```python
from build123d import *

# Parameters (mm, degrees)
SKETCH1_W           = 60
SKETCH1_H           = 27
BOSS_EXTRUDE1_DEPTH = 10
SKETCH2_R           = 2.6
CUT_EXTRUDE1_DEPTH  = 42.581245773
SKETCH3_R           = 4.75
CUT_EXTRUDE2_DEPTH  = 22
SKETCH4_W           = 60
SKETCH4_H           = 7
SKETCH4_W_2         = 40
SKETCH4_H_2         = 5
BOSS_EXTRUDE3_DEPTH = 28
SKETCH5_R           = 2.6
CUT_EXTRUDE3_DEPTH  = 50.122296363
SKETCH6_R           = 1.6
CUT_EXTRUDE4_DEPTH  = 51.261814532


with BuildPart() as part:
    # Sketch1 → Boss-Extrude1 (new body)
    with BuildSketch(Plane(origin=(0, 0, 0), x_dir=(1, 0, 0), z_dir=(0, 1, 0))):
        Rectangle(SKETCH1_W, SKETCH1_H)
    extrude(amount=BOSS_EXTRUDE1_DEPTH)

    # Sketch2 → Cut-Extrude1 (cut, through all)
    with BuildSketch(Plane.XY.offset(13.5)):
        with Locations((0, 5)):
            Circle(SKETCH2_R)
    extrude(amount=-CUT_EXTRUDE1_DEPTH, mode=Mode.SUBTRACT)

    # Sketch3 → Cut-Extrude2 (cut)
    with BuildSketch(Plane.XY.offset(13.5)):
        with Locations((0, 5)):
            Circle(SKETCH3_R)
    extrude(amount=-CUT_EXTRUDE2_DEPTH, mode=Mode.SUBTRACT)

    # Sketch4 → Boss-Extrude3 (add)
    with BuildSketch(Plane.XZ):
        with Locations((0, 10)):
            Rectangle(SKETCH4_W, SKETCH4_H)
        with Locations((0, 10)):
            Rectangle(SKETCH4_W_2, SKETCH4_H_2, mode=Mode.SUBTRACT)
    extrude(amount=BOSS_EXTRUDE3_DEPTH)

    # Sketch5 → Cut-Extrude3 (cut, through all)
    with BuildSketch(Plane.XY.offset(13.5)):
        with Locations((0, -22.5)):
            Circle(SKETCH5_R)
    extrude(amount=-CUT_EXTRUDE3_DEPTH, mode=Mode.SUBTRACT)

    # Sketch6 → Cut-Extrude4 (cut, through all)
    with BuildSketch(Plane(origin=(0, 10, 0), x_dir=(1, 0, 0), z_dir=(0, 1, 0))):
        with Locations(Location((-10, -10, 0), (0, 0, 270))):
            Circle(SKETCH6_R)
        with Locations(Location((10, -10, 0), (0, 0, 270))):
            Circle(SKETCH6_R)
    extrude(amount=-CUT_EXTRUDE4_DEPTH, mode=Mode.SUBTRACT)


solid = part.part
```
Check sheet for the modelled part. Datum: model origin and axes. Units: mm. A direction names the side the tool comes from. Round coordinates to 2 decimals unless told otherwise and drop trailing zeros. Write each loop counter-clockwise with the first axis right and the second up, starting at its lowest first coordinate (ties: lowest second). Pieces come first, ordered by that corner, then holes. Notation, with made-up numbers: (-18, 43) -> (-14, 43) arc R27 cw to (-14, 72) -> close; hole circle Ø11 at (63, 47). An arc over 180 degrees is marked (long way). Put each result on its own line as item: value.
(1) Sectioned sample at A-A (z = 10). Enter the section's corners in (x, y), plus the area to 3 significant figures.
Values found:
outline: (-30, -28) -> (-20, -28) -> (-20, 0) -> (-11.6, 0) -> (-11.6, 10) -> (-30, 10) -> close; (-8.4, 0) -> (8.4, 0) -> (8.4, 10) -> (-8.4, 10) -> close; (11.6, 0) -> (20, 0) -> (20, -28) -> (30, -28) -> (30, 10) -> (11.6, 10) -> close; hole circle Ø9.5 at (0, 5)
area: 1,030 mm^2
(2) Go/stop test with flat-tipped pins: pin 1 Ø7.5 at (x, y) = (0, 5) entering from +Z; pin 2 Ø10 at (x, y) = (12.5, -7) entering from -Z; pin 3 Ø10 at (x, z) = (-8, -7) entering from -Y. Record where each tip stops, or that it passes through.
Values found:
pin 1: stops at z = -8.5
pin 2: stops at z = 6.5
pin 3: stops at y = 0
(3) Sectioned sample at C-C (y = -16.5). Enter the section's corners in (x, z).
Values found:
outline: (-30, 6.5) -> (30, 6.5) -> (30, 13.5) -> (-30, 13.5) -> close; hole (-20, 7.5) -> (20, 7.5) -> (20, 12.5) -> (-20, 12.5) -> close
(4) Sectioned sample at D-D (x = 10). Enter the section's corners in (y, z).
Values found:
outline: (-28, 6.5) -> (0, 6.5) -> (0, -13.5) -> (10, -13.5) -> (10, 8.4) -> (0, 8.4) -> (0, 7.5) -> (-28, 7.5) -> close; (-28, 12.5) -> (0, 12.5) -> (0, 11.6) -> (10, 11.6) -> (10, 13.5) -> (-28, 13.5) -> close
(5) Tool access check on faces 1 (the face through (30, 0, 9)), 2 (the face through (0, 0, -4)), 3 (the face through (2, 3, -8.5)), 4 (the face through (0, 0, 10)), 5 (the face through (0, 2, -13.5)). Record the directions out of +Z, -Z, +X, -X, +Y, -Y that give a thin tool (end or side, any length) a straight path to the whole face; none if there is none.
Values found:
face 1: +Z, -Z, +X, +Y, -Y
face 2: -Z, +X, -X, -Y
face 3: +Z
face 4: -Y
face 5: -Z, +X, -X, +Y, -Y
(6) Sectioned sample at B-B (y = 5). Enter the section's corners in (x, z).
Values found:
outline: (-30, -13.5) -> (-2.6, -13.5) -> (-2.6, -8.5) -> (-4.75, -8.5) -> (-4.75, 13.5) -> (-30, 13.5) -> close; (2.6, -13.5) -> (30, -13.5) -> (30, 13.5) -> (4.75, 13.5) -> (4.75, -8.5) -> (2.6, -8.5) -> close; hole circle Ø3.2 at (-10, 10); hole circle Ø3.2 at (10, 10)
(7) Mould release check, pull along Y, two halves, no side actions. Record for faces 6 (the face through (-30, 0, 9)), 7 (the face through (2.554, 9.005, 2.654)), 8 (the face through (0, 10, 0)): released by +Y, released by -Y, zero draft, split by the parting line, or undercut.
Values found:
face 6: zero draft
face 7: undercut
face 8: released by +Y
(8) Material ranges on line 1 (Y direction, x = 0, z = 6.7); line 2 (Y direction, x = 0, z = -11.4); line 3 (Y direction, x = 0, z = -2.25), recorded low to high.
Values found:
line 1: y = -28 to -25.1, -19.9 to 0.25, 9.75 to 10
line 2: y = 0 to 2.4, 7.6 to 10
line 3: y = 0 to 0.25, 9.75 to 10
